from build123d import *

# Parameters (mm, degrees)
PAD_DEPTH              = 3
PAD001_DEPTH           = 7
PAD002_DEPTH           = 18
SKETCH003_W            = 1
SKETCH003_H            = 10.328695
POCKET_DEPTH           = 1
LINEARPATTERN_COUNT    = 4
LINEARPATTERN_PITCH    = 20
LINEARPATTERN001_COUNT = 4
LINEARPATTERN001_PITCH = 20
LINEARPATTERN002_COUNT = 4
LINEARPATTERN002_PITCH = 20
CHAMFER_SIZE           = 1
CHAMFER001_SIZE        = 0.8
CHAMFER002_SIZE        = 1


with BuildPart() as part:
    # Sketch → Pad (new body)
    with BuildSketch(Plane.XY):
        with BuildLine():
            Line((-34, 15), (34, 15))
            ThreePointArc((40, 9), (38.242641, 13.242641), (34, 15))
            Line((40, 9), (40, -4))
            ThreePointArc((34, -10), (38.242641, -8.242641), (40, -4))
            Line((34, -10), (-34, -10))
            ThreePointArc((-40, -4), (-38.242641, -8.242641), (-34, -10))
            Line((-40, -4), (-40, 9))
            ThreePointArc((-34, 15), (-38.242641, 13.242641), (-40, 9))
        make_face()
    extrude(amount=PAD_DEPTH)

    # Sketch001 (on Face10 of Pad) → Pad001 (join)
    with BuildSketch(Plane.XY.offset(3)):
        with BuildLine():
            Line((-32.071835, -2.1), (-27.928165, -2.1))
            ThreePointArc((-27.928165, -2.1), (-30, 2.95), (-32.071835, -2.1))
        make_face()
    pad001 = extrude(amount=PAD001_DEPTH)

    # Sketch002 (on Face5 of Pad001) → Pad002 (join)
    with BuildSketch(Plane.XY.offset(3)):
        with BuildLine():
            ThreePointArc((-26.888889, 6.270645), (-30, 7), (-33.111111, 6.270645))
            ThreePointArc((-34.888889, 9.853871), (-35.791613, 7.173369), (-33.111111, 6.270645))
            ThreePointArc((-25.111111, 9.853871), (-30, 11), (-34.888889, 9.853871))
            ThreePointArc((-26.888889, 6.270645), (-24.208387, 7.173369), (-25.111111, 9.853871))
        make_face()
    pad002 = extrude(amount=PAD002_DEPTH)

    # Sketch003 (on Face18 of Pad002) → Pocket (cut)
    with BuildSketch(Plane.XY.offset(21)):
        with Locations((-30, 9.690067)):
            Rectangle(SKETCH003_W, SKETCH003_H)
    pocket = extrude(amount=-POCKET_DEPTH, mode=Mode.SUBTRACT)

    # LinearPattern: Pad001 ×4
    with Locations(*[(i * LINEARPATTERN_PITCH, 0, 0) for i in range(1, LINEARPATTERN_COUNT)]):
        add(pad001)

    # LinearPattern001: Pad002 ×4
    with Locations(*[(i * LINEARPATTERN001_PITCH, 0, 0) for i in range(1, LINEARPATTERN001_COUNT)]):
        add(pad002)

    # LinearPattern002: Pocket ×4
    with Locations(*[(i * LINEARPATTERN002_PITCH, 0, 0) for i in range(1, LINEARPATTERN002_COUNT)]):
        add(pocket, mode=Mode.SUBTRACT)

    # Chamfer
    chamfer_edges = [part.edges().sort_by_distance(p)[0] for p in [
        (-40, 2.5, 3),
        (-38.242641, -8.242641, 3),
        (-38.242641, 13.242641, 3),
        (0, -10, 3),
        (0, 15, 3),
        (38.242641, -8.242641, 3),
        (38.242641, 13.242641, 3),
        (40, 2.5, 3),
        (10, 7, 3),
        (15.791613, 7.173369, 3),
        (4.208387, 7.173369, 3),
        (10, 11, 3),
        (-10, 7, 3),
        (-4.208387, 7.173369, 3),
        (-15.791613, 7.173369, 3),
        (-10, 11, 3),
        (-30, 7, 3),
        (-24.208387, 7.173369, 3),
        (-35.791613, 7.173369, 3),
        (-30, 11, 3),
        (-30, 2.95, 3),
        (-30, -2.1, 3),
        (30, 2.95, 3),
        (30, -2.1, 3),
        (30, 7, 3),
        (24.208387, 7.173369, 3),
        (30, 11, 3),
        (35.791613, 7.173369, 3),
        (-10, 2.95, 3),
        (-10, -2.1, 3),
        (10, 2.95, 3),
        (10, -2.1, 3),
        (-40, 2.5, 0),
        (-38.242641, 13.242641, 0),
        (0, 15, 0),
        (38.242641, 13.242641, 0),
        (40, 2.5, 0),
        (38.242641, -8.242641, 0),
        (0, -10, 0),
        (-38.242641, -8.242641, 0),
    ]]
    chamfer(chamfer_edges, length=CHAMFER_SIZE)

    # Chamfer001
    chamfer001_edges = [part.edges().sort_by_distance(p)[0] for p in [
        (-30, -2.1, 10),
        (-30, 2.95, 10),
        (-10, -2.1, 10),
        (-10, 2.95, 10),
        (10, -2.1, 10),
        (10, 2.95, 10),
        (30, -2.1, 10),
        (30, 2.95, 10),
    ]]
    chamfer(chamfer001_edges, length=CHAMFER001_SIZE)

    # Chamfer002
    chamfer002_edges = [part.edges().sort_by_distance(p)[0] for p in [
        (-35.791613, 7.173369, 21),
        (-24.208387, 7.173369, 21),
        (-15.791613, 7.173369, 21),
        (-4.208387, 7.173369, 21),
        (4.208387, 7.173369, 21),
        (15.791613, 7.173369, 21),
        (24.208387, 7.173369, 21),
        (35.791613, 7.173369, 21),
    ]]
    chamfer(chamfer002_edges, length=CHAMFER002_SIZE)


solid = part.part
For this review, take the finished solid that the model builds, in its own axes (mm). A direction names the side the tool comes from. Round coordinates to 2 decimals unless told otherwise and drop trailing zeros. Write each loop counter-clockwise with the first axis right and the second up, starting at its lowest first coordinate (ties: lowest second). Pieces come first, ordered by that corner, then holes. Notation, with made-up numbers: M 64.25,32.25 L 107.25,32.25 A11 ccw 107.25,45.25 Z; hole C 40,66 d9. An arc over 180 degrees is marked long. Write item = value, one per line. Start each with the question number.
(1) For line 1 along Y through (x, z) = (-30, 6.75); line 2 along Z through (x, y) = (-0.5, 3); line 3 along Y through (x, z) = (-9.5, 16.25), list the stretches that pass through material, from the lowest coordinate up.
(2) Clearance check with flat-ended pins moving along their axes: pin 1 Ø0.5 at (x, y) = (-10, 9) entering from +Z; pin 2 Ø2 at (x, z) = (-15, 8.5) entering from +Y; pin 3 Ø0.8 at (y, z) = (8.5, 20.5) entering from -X. State where each tip first meets the part, or that it passes through.
(3) The part is to be moulded in two halves that separate along Y. For faces 1 (the face through (-10, 0, 10)), 2 (the face through (37.778, -7.696, 2.715)), 3 (the face through (10.08, 2.28, 9.87)), say which applies: +Y half, -Y half, draft (parallel to the pull), parting line (faces both ways), or undercut.
(4) For faces 4 (the face through (-10, 11, 12)), 5 (the face through (-30, -2.1, 7)), 6 (the face through (1, 3, 3)), 7 (the face through (-13, 9, 21)), list the 3-axis set-ups (+Z, -Z, +X, -X, +Y, -Y) from which the entire face can be reached by the end or side of a thin tool; tool diameter is ignored.
(5) We need section A-A (x = 18). Give the boundary of the cut face in (y, z).
Results found:
q1.line_1 = -2.1 to 2.95, 7 to 11
q1.line_2 = 0 to 3
q1.line_3 = 6.98 to 10.99
q2.pin_1 = 20
q2.pin_2 = 10.25
q2.pin_3 = -35.86
q3.face_1 = draft
q3.face_2 = -Y half
q3.face_3 = undercut
q4.face_4 = +Z, +Y
q4.face_5 = +Z, +X, -X, -Y
q4.face_6 = +Z
q4.face_7 = +Z, +X, -X, +Y, -Y
q5.outline = M -10,1 L -9,0 L 14,0 L 15,1 L 15,2 L 14,3 L -9,3 L -10,2 Z
